```python
from build123d import *

# Parameters (mm, degrees)
F2_SIZE = 4


# Not quite as in the source:
# - a fillet or chamfer that OpenCascade refuses, or shapes differently, is made with other operations: its cross-section is extruded or revolved along the edge and cut away or added


with BuildPart() as f1:
    # F0 (on Front) → F1 (revolve)
    with BuildSketch(Plane.XZ):
        with BuildLine():
            Line((-55, 0), (-55, 7.5))
            Line((-55, 7.5), (55, 7.5))
            Line((55, 7.5), (55, 15.5))
            Line((55, 15.5), (50, 15.5))
            Line((50, 15.5), (50, 13.5))
            Line((50, 13.5), (49.3, 13.5))
            Line((49.3, 13.5), (49.3, 15.5))
            ThreePointArc((49.3, 15.5), (47.8, 17), (46.3, 15.5))
            Line((46.3, 15.5), (46.3, 14))
            Line((46.3, 14), (-50.3, 14))
            Line((-50.3, 14), (-50.3, 15.5))
            ThreePointArc((-50.3, 15.5), (-51.8, 17.0770088649), (-53.3, 15.5))
            Line((-53.3, 15.5), (-53.3, 13.5))
            Line((-53.3, 13.5), (-54, 13.5))
            Line((-54, 13.5), (-54, 15.5))
            Line((-54, 15.5), (-59, 15.5))
            Line((-59, 15.5), (-59, 0))
            Line((-59, 0), (-55, 0))
        make_face()
    revolve(axis=Axis((-4.5135766268, 0, 0), (1, 0, 0)))

    # F2
    f2_edges = [f1.edges().sort_by_distance(p)[0] for p in [
        (55, 0, -7.5),
    ]]
    chamfer(f2_edges, length=F2_SIZE)

    # F3: chamfer of 0.5 on 5 edges, made by hand

    # F3_s1 → F3_t2 (revolve, cut)
    with BuildSketch(Plane.XZ):
        Polygon((55, 15), (54.5, 15.5), (55, 15.5), align=None)
    revolve(axis=Axis((55, 0, 0), (1, 0, 0)), mode=Mode.SUBTRACT)

    # F3_s3 → F3_t4 (revolve, cut)
    with BuildSketch(Plane.XZ):
        Polygon((54.8535533906, 11.3535533906), (55, 11.7071067812), (55, 11.5), align=None)
    revolve(axis=Axis((55, 0, 0), (1, 0, 0)), mode=Mode.SUBTRACT)

    # F3_s5 → F3_t6 (revolve, cut)
    with BuildSketch(Plane.XZ):
        Polygon((-58.5, 15.5), (-59, 15), (-59, 15.5), align=None)
    revolve(axis=Axis((-59, 0, 0), (1, 0, 0)), mode=Mode.SUBTRACT)

    # F3_s7 → F3_t8 (revolve, cut)
    with BuildSketch(Plane.XZ):
        Polygon((-54, 15), (-54.5, 15.5), (-54, 15.5), align=None)
    revolve(axis=Axis((-54, 0, 0), (1, 0, 0)), mode=Mode.SUBTRACT)

    # F3_s9 → F3_t10 (revolve, cut)
    with BuildSketch(Plane.XZ):
        Polygon((50.5, 15.5), (50, 15), (50, 15.5), align=None)
    revolve(axis=Axis((50, 0, 0), (1, 0, 0)), mode=Mode.SUBTRACT)


solid = f1.part
```
Verification items for the finished model (mm, model axes). A direction names the side the tool comes from. Round coordinates to 2 decimals unless told otherwise and drop trailing zeros. Write each loop counter-clockwise with the first axis right and the second up, starting at its lowest first coordinate (ties: lowest second). Pieces come first, ordered by that corner, then holes. Notation, with made-up numbers: (12, 21.5) - (54, 21.5) arc R21 ccw to (54, 46.5) - close; hole circle Ø5 at (68, 53.25). An arc over 180 degrees is marked (long way). Answer as a JSON object with one key per item and string values. Group by question number.
Q1. Thickness scan on line 1 (Z direction, x = 28, y = 0); line 2 (X direction, y = -13, z = 8.5). Record the ranges inside material, lowest first.
Q2. Mould release check, pull along X, two halves, no side actions. Record for faces 1 (the cylindrical face through (-56.528, -15.368, -2.018)), 2 (the flat face through (-59, 0, 0)), 3 (the flat face through (50, -7.85, -11.18)), 4 (the flat face through (-55, 0, 0)): released by +X, released by -X, zero draft, split by the parting line, or undercut.
Q3. Section check A-A, the plane x = -35.5. Enter the section's corners in (y, z), plus the area to 3 significant figures.
Q4. Go/stop test with flat-tipped pins: pin 1 Ø5 at (x, y) = (7, 11) entering from +Z; pin 2 Ø6 at (x, y) = (24, 13.5) entering from -Z; pin 3 Ø8 at (x, y) = (10.5, 7) entering from -Z. Record where each tip stops, or that it passes through.
Q5. Tool access check on faces 5 (the cylindrical face through (-1.258, -0.33, -7.493)), 6 (the cylindrical face through (-53.65, 13.18, -2.93)). Record the directions out of +Z, -Z, +X, -X, +Y, -Y that give a thin tool (end or side, any length) a straight path to the whole face; none if there is none.
Found:
{
 "1": {"line 1": "z = -14 to -7.5, 7.5 to 14", "line 2": "x = -53.3 to -50.3, 46.3 to 49.3"},
 "2": {"face 1": "zero draft", "face 2": "released by -X", "face 3": "undercut", "face 4": "released by +X"},
 "3": {"outline": "circle Ø28 at (0, 0); hole circle Ø15 at (0, 0)", "area": "439 mm^2"},
 "4": {"pin 1": "stops at z = 11.12", "pin 2": "stops at z = -9.26", "pin 3": "stops at z = -13.67"},
 "5": {"face 5": "+X", "face 6": "none"}
}
